Read the model definition and answer for the solid it produces. Units are mm, in the model's axes. A direction names the side the tool comes from. Give positions to 0.01 mm unless a question says otherwise; leave off trailing zeros. Loops run counter-clockwise (first coordinate to the right, second up) from the corner with the lowest first, then second, coordinate; pieces in that order, holes last.
(1) Each of these flat-tipped pins is pushed along its axis until it touches: P1, Ø12, axis at x = 2.5, z = 82, coming from the +Y side; P2, Ø24.5, axis at x = -3, y = -0.5, coming from the +Z side; P3, Ø10, axis at y = 22.5, z = 50.5, coming from the -X side; P4, Ø12, axis at x = -63.5, y = 3.5, coming from the +Z side. Where does it stop, or does it pass through?
(2) Determine the mould class of faces 1 (the face through (12.4, 2.75, 59.48)), 2 (the face through (-38.393, -1.907, 18.783)), 3 (the face through (-1, 19, 0)), 4 (the face through (-79.375, 1, 19)) for opening direction X: pulls with the +X half, pulls with the -X half, needs draft (parallel to the pull), parting line crosses it, or undercut.
(3) Find section A-A, the plane y = 0. Write down the section's boundary in (x, z) (3 decimals), then the cut area to 3 significant figures.
(4) Which of the six approach directions +Z, -Z, +X, -X, +Y, -Y give full straight-line access (tool end or side, diameter ignored) to faces 5 (the face through (11, -11, 133.35)), 6 (the face through (14.88, 3.3, 126.91))?
(5) Straight lines are drawn through the part: probe 1 along X at (y, z) = (44, 11) (3 decimals); probe 2 along X at (y, z) = (0.5, 76); probe 3 along Y at (x, z) = (0, 96). For each, find the intervals that lie inside material, in ascending order.
(6) Find section C-C, the plane z = 14.5. Write down the section's boundary in (x, y) (3 decimals).
(7) Find section D-D, the plane x = -46. Write down the section's boundary in (y, z) (3 decimals), then the cut area to 3 significant figures.
Autodesk Inventor part; units mm, degrees
ref_plane "YZ Plane" through (0, 0, 0) normal (1, 0, 0) x (0, 1, 0)
ref_plane "XZ Plane" through (0, 0, 0) normal (0, 1, 0) x (-1, 0, 0)
ref_plane "XY Plane" through (0, 0, 0) normal (0, 0, 1) x (1, 0, 0)
ref_plane "Work Plane1" through (0, 0, 0) normal (0, 0, 1) x (1, 0, 0)
sketch "Sketch1" plane through (0, 0, 0) normal (0, 0, 1) x (1, 0, 0)
  line L0 (79.375, 79.375) -> (-79.375, 79.375)
  line L1 (-79.375, 79.375) -> (-79.375, -79.375)
  line L2 (-79.375, -79.375) -> (79.375, -79.375)
  line L3 (79.375, -79.375) -> (79.375, 79.375)
  line L4 (79.375, 79.375) -> (-79.375, -79.375) construction
  line L5 (-79.375, 79.375) -> (79.375, -79.375) construction
  point P0 (0, 0)
  dimension "d0" = 158.75
  dimension "d1" = 158.75
extrude "Extrusion1" add sketch "Sketch1" along normal blind 38.1
sketch "Sketch2" plane through (0, 0, 38.1) normal (0, 0, 1) x (1, 0, 0)
  circle A0 centre (0, 0) radius 25.4
  dimension "d4" = 50.8
extrude "Extrusion2" add sketch "Sketch2" along normal blind 95.25
hole "Hole1" at (0, 0, 133.35) direction (0, 0, -1) diameter 25.4 end through all counterbore diameter 30.48 counterbore depth 12.7
sketch "Sketch3" plane through (0, 0, 38.1) normal (0, 0, 1) x (1, 0, 0)
  circle A0 centre (0, 0) radius 12.7 construction
  circle A1 centre (0, 0) radius 44.45 construction
  point P0 (0, 44.45)
  dimension "d16" = 88.9
hole "Hole2" at (0, 44.45, 38.1) direction (0, 0, -1) diameter 12.7 end through all
pattern_circular "Circular Pattern1" count 4 over 360 about axis through (0, 0, 38.1) along (0, 0, 1) of "Hole2"
properties part number "Base"
Entries:
1. P1: stops at y = 25.4
1. P2: stops at z = 133.35
1. P3: stops at x = -18.41
1. P4: stops at z = 38.1
2. face 1: undercut
2. face 2: undercut
2. face 3: needs draft
2. face 4: pulls with the -X half
3. outline: (-79.375, 0) - (-50.8, 0) - (-50.8, 38.1) - (-79.375, 38.1) - close; (-38.1, 0) - (-12.7, 0) - (-12.7, 120.65) - (-15.24, 120.65) - (-15.24, 133.35) - (-25.4, 133.35) - (-25.4, 38.1) - (-38.1, 38.1) - close; (12.7, 0) - (38.1, 0) - (38.1, 38.1) - (25.4, 38.1) - (25.4, 133.35) - (15.24, 133.35) - (15.24, 120.65) - (12.7, 120.65) - close; (50.8, 0) - (79.375, 0) - (79.375, 38.1) - (50.8, 38.1) - close
3. area: 6,470 mm2
4. face 5: +Z, +X, -X, +Y, -Y
4. face 6: +Z
5. probe 1: x = -79.375 to -6.334, 6.334 to 79.375
5. probe 2: x = -25.4 to -12.69, 12.69 to 25.4
5. probe 3: y = -25.4 to -12.7, 12.7 to 25.4
6. outline: (-79.375, -79.375) - (79.375, -79.375) - (79.375, 79.375) - (-79.375, 79.375) - close; hole circle Ø12.7 at (-44.45, 0); hole circle Ø25.4 at (0, 0); hole circle Ø12.7 at (0, -44.45); hole circle Ø12.7 at (0, 44.45); hole circle Ø12.7 at (44.45, 0)
7. outline: (-79.375, 0) - (-6.158, 0) - (-6.158, 38.1) - (-79.375, 38.1) - close; (6.158, 0) - (79.375, 0) - (79.375, 38.1) - (6.158, 38.1) - close
7. area: 5,580 mm2
